from build123d import *

# Parameters (mm, degrees)
F0_R     = 12.7
F1_DEPTH = 25.4
F2_R     = 6.35
F3_R     = 6.35
F4_DEPTH = 25.4


with BuildPart() as f1:
    # F0 (on Top) → F1 (new body)
    with BuildSketch(Plane.XY):
        Circle(F0_R)
    extrude(amount=F1_DEPTH)

    # F2
    f2_edges = [f1.edges().sort_by_distance(p)[0] for p in [
        (12.7, 0, 12.7),
        (-12.7, 0, 0),
        (-12.7, 0, 25.4),
    ]]
    fillet(f2_edges, radius=F2_R)

    # F3 (on Top) → F4 (cut)
    with BuildSketch(Plane.XY):
        Circle(F3_R)
    extrude(amount=F4_DEPTH, mode=Mode.SUBTRACT)


solid = f1.part
The listing builds one solid part. Answer for the finished solid, in the listing's coordinates (mm). Round coordinates to 2 decimals unless told otherwise and drop trailing zeros. Answer in a Markdown table with one row per item. Add a question column.
1) Determine the mould class of faces 1 (the face through (-1.38, -6.2, 12.52)), 2 (the face through (-2.75, -12.4, 12.61)) for opening direction X: pulls with the +X half, pulls with the -X half, needs draft (parallel to the pull), parting line crosses it, or undercut.
2) Consider line 1 along Y through (x, z) = (0, 8); line 2 along Y through (x, z) = (-4.75, 18); line 3 along X through (y, z) = (2.5, 18). Determine where each line is inside the solid, lowest interval first. Write a range as from..to.
3) Flat-ended cylindrical pins translate along their axes: pin 1 Ø8 at (y, z) = (-6.5, 7) entering from +X; pin 2 Ø5 at (x, z) = (-5.5, 7) entering from +Y; pin 3 Ø2 at (y, z) = (-6, 10.5) entering from +X; pin 4 Ø6 at (x, y) = (5, 6) entering from +Z. Find the tip coordinate at first contact, or state that the pin passes through.
Findings below:
| question | item | result |
|---|---|---|
| 1 | face 1 | undercut |
| 1 | face 2 | parting line crosses it |
| 2 | line 1 | y = -12.7..-6.35, 6.35..12.7 |
| 2 | line 2 | y = -11.78..-4.21, 4.21..11.78 |
| 2 | line 3 | x = -12.45..-5.84, 5.84..12.45 |
| 3 | pin 1 | stops at x = 12.45 |
| 3 | pin 2 | stops at y = 12.34 |
| 3 | pin 3 | stops at x = 11.67 |
| 3 | pin 4 | stops at z = 25.4 |
